```python
from build123d import *

# Parameters (mm, degrees)
F1_DEPTH = 30
F2_SIZE  = 7.5
F4_DEPTH = 299.001
F5_SIZE  = 5
F6_R     = 2.5
F7_DEPTH = 179.001
F8_R     = 2.5
F9_DEPTH = 15.001
F10_SIZE = 2.5


with BuildPart() as f1:
    # F0 (on Front) → F1 (new body)
    with BuildSketch(Plane.XZ):
        Polygon((-149.5, 0), (0, 0), (149.5, 0), (149.5, 15), (29.5, 15), (29.5, 45), (19.5, 45), (19.5, 15), (0, 15), (-19.5, 15), (-19.5, 45), (-29.5, 45), (-29.5, 15), (-149.5, 15), align=None)
    extrude(amount=F1_DEPTH)

    # F2
    f2_edges = [f1.edges().sort_by_distance(p)[0] for p in [
        (-89.5, -30, 15),
        (-89.5, 0, 15),
        (89.5, 0, 15),
        (89.5, -30, 15),
    ]]
    chamfer(f2_edges, length=F2_SIZE)

    # F3 (on face) → F4 (cut, through all)
    with BuildSketch(Plane(origin=(-149.5, 0, 0), x_dir=(0, -1, 0), z_dir=(-1, 0, 0))):
        Polygon((5.000000033, 5.4289321745), (5.000000033, 0), (24.999999967, 0), (24.999999967, 5.4289321745), (20.4289321745, 9.999999967), (9.5710678255, 9.999999967), align=None)
    extrude(amount=-F4_DEPTH, mode=Mode.SUBTRACT)

    # F5
    f5_edges = [f1.edges().sort_by_distance(p)[0] for p in [
        (-24.5, 0, 45),
        (-24.5, -30, 45),
        (24.5, 0, 45),
        (24.5, -30, 45),
    ]]
    chamfer(f5_edges, length=F5_SIZE)

    # F6 (on face) → F7 (cut, through all)
    with BuildSketch(Plane.YZ.offset(29.5)):
        with Locations((-15, 35)):
            Circle(F6_R)
    extrude(amount=-F7_DEPTH, mode=Mode.SUBTRACT)

    # F8 (on face) → F9 (cut, through all)
    with BuildSketch(Plane.XY.offset(15)):
        with Locations((0, -15)):
            Circle(F8_R)
    extrude(amount=-F9_DEPTH, mode=Mode.SUBTRACT)

    # F10
    f10_edges = [f1.edges().sort_by_distance(p)[0] for p in [
        (-29.5, -17.5, 35),
        (29.5, -17.5, 35),
        (-2.5, -15, 10),
    ]]
    chamfer(f10_edges, length=F10_SIZE)


solid = f1.part
```
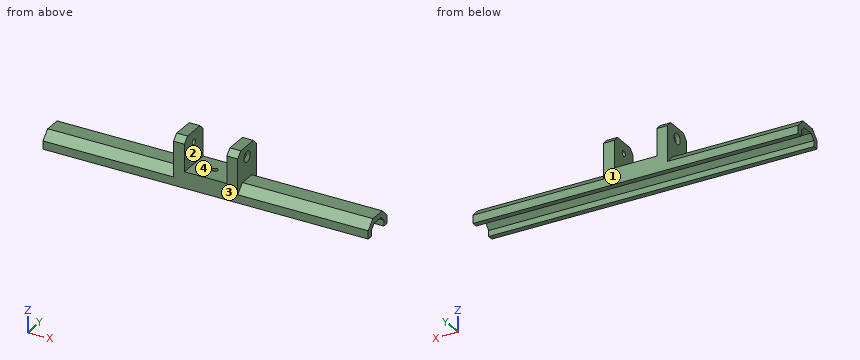
Source: CAD feature listing. Evaluate the final solid. Frame: model axes, mm. Face numbers are marked on the shaded views. A direction names the side the tool comes from. Give positions to 0.01 mm unless a question says otherwise; leave off trailing zeros. Loops run counter-clockwise (first coordinate to the right, second up) from the corner with the lowest first, then second, coordinate; pieces in that order, holes last. Notation, with made-up numbers: (-33.5, 12) -> (19.5, 12) arc R24 cw to (19.5, 43) -> close; hole circle Ø8 at (54.25, 11). An arc over 180 degrees is marked (long way). Put each result on its own line as item: value. Start each with the question number.
1) Contact query for flat-ended pins moving along their axis: P1, Ø1.5, axis at x = -96.5, y = -19.5, coming from the -Z side; P2, Ø12, axis at x = 100, y = -13.5, coming from the +Z side; P3, Ø15, axis at y = -17, z = 23, coming from the -X side. Output: stop coordinate, or through.
2) Cut plane B-B (z = 42.5). Return loops of the section in (x, y), then the cut area to 3 significant figures.
3) Reachability of the marked faces 3 and 4 from +Z, -Z, +X, -X, +Y, -Y: full face, straight path, thin tool, end or side. Return the list, or none.
4) Cut plane D-D (x = 59.5). Return loops of the section in (y, z).
5) Cut plane A-A (y = -15). State how many separate pieces and enclosed holes the cut face has, then the cut area to 3 significant figures.
6) Cut plane C-C (x = 0). Return loops of the section in (y, z), then the cut area to 3 significant figures.
7) Draft query along X for the marked faces 1 and 2. Return one class per face: released by +X, released by -X, zero draft, split by the parting line, or undercut.
8) Material intervals for probe 1 along Y at (x, z) = (0, 13); probe 2 along X at (y, z) = (-24, 40.5); probe 3 along Y at (x, z) = (25, 5), sorted ascending.
Results are:
1. P1: stops at z = 10
1. P2: stops at z = 15
1. P3: stops at x = -29.5
2. outline: (-29.5, -27.5) -> (-19.5, -27.5) -> (-19.5, -2.5) -> (-29.5, -2.5) -> close; (19.5, -27.5) -> (29.5, -27.5) -> (29.5, -2.5) -> (19.5, -2.5) -> close
2. area: 500 mm2
3. face 3: +Z, -Z, +X, -X, -Y
3. face 4: +Z, +Y, -Y
4. outline: (-30, 0) -> (-25, 0) -> (-25, 5.43) -> (-20.43, 10) -> (-9.57, 10) -> (-5, 5.43) -> (-5, 0) -> (0, 0) -> (0, 7.5) -> (-7.5, 15) -> (-22.5, 15) -> (-30, 7.5) -> close
5. separate pieces: 4
5. enclosed holes: 0
5. area: 1,950 mm2
6. outline: (-30, 0) -> (-25, 0) -> (-25, 5.43) -> (-20.43, 10) -> (-20, 10) -> (-17.5, 12.5) -> (-17.5, 15) -> (-30, 15) -> close; (-12.5, 12.5) -> (-10, 10) -> (-9.57, 10) -> (-5, 5.43) -> (-5, 0) -> (0, 0) -> (0, 15) -> (-12.5, 15) -> close
6. area: 240 mm2
7. face 1: zero draft
7. face 2: undercut
8. probe 1: y = -30 to -17.5, -12.5 to 0
8. probe 2: x = -29.5 to -19.5, 19.5 to 29.5
8. probe 3: y = -30 to -25, -5 to 0
